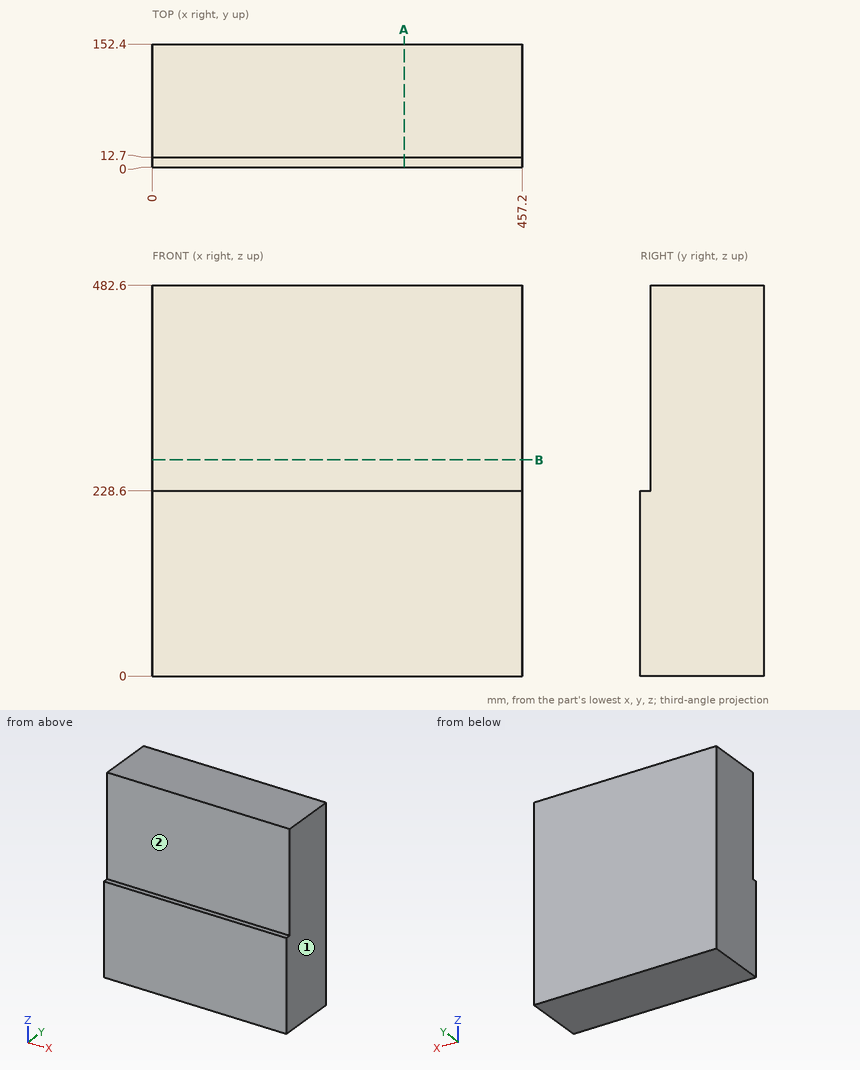
Here's the drawing with two shaded views (mm, measured from the low corner). I have some questions. A direction names the side the tool comes from. Round coordinates to 2 decimals unless told otherwise and drop trailing zeros. Write each loop counter-clockwise with the first axis right and the second up, starting at its lowest first coordinate (ties: lowest second). Pieces come first, ordered by that corner, then holes.
(1) Suppose I cut it at A-A on x = 311. Write out the boundary of the cut face in (y, z).
Findings below:
outline: (0, 0) - (152.4, 0) - (152.4, 482.6) - (12.7, 482.6) - (12.7, 228.6) - (0, 228.6) - close
(2) Suppose I cut it at B-B on z = 267. Write out the boundary of the cut face in (x, y).
Findings below:
outline: (0, 12.7) - (457.2, 12.7) - (457.2, 152.4) - (0, 152.4) - close
(3) If I drill on probe 1 along Y at (x, z) = (359, 436); probe 2 along Z at (x, y) = (383, 7), over which ranges is the centre line in solid material (lowest first)?
Findings below:
probe 1: y = 12.7 to 152.4
probe 2: z = 0 to 228.6
(4) For pin 1 (1 mm diameter, centred on x = 286, z = 383.5, fed in from -Y); pin 2 (4 mm diameter, centred on x = 323, y = 4, fed in from +Z), each with a flat end and sliding along its axis, tell me the tip position at first contact or that it passes through.
Findings below:
pin 1: stops at y = 12.7
pin 2: stops at z = 228.6
(5) Which directions (+Z, -Z, +X, -X, +Y, -Y) give clear straight access to the entire face, cutting with the end or side of a thin tool? Please do the marked faces 1 and 2.
Findings below:
face 1: +Z, -Z, +X, +Y, -Y
face 2: +Z, +X, -X, -Y
